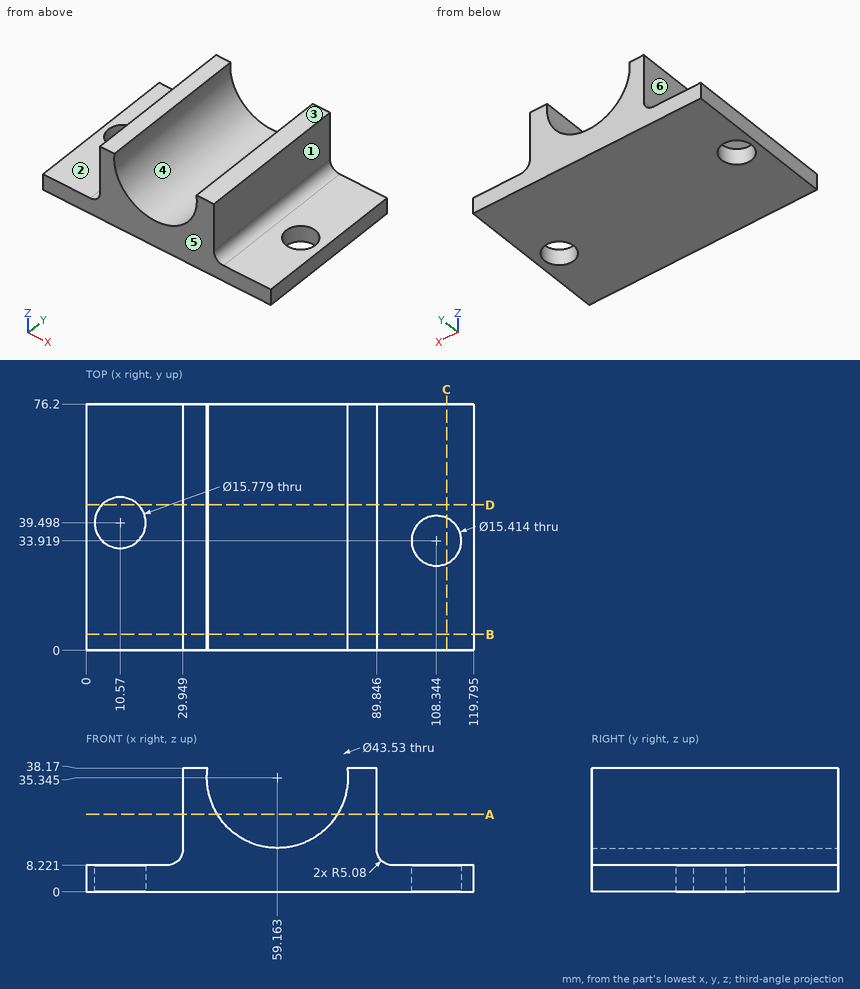
Study the drawing (mm; zero at the part's minimum x, y, z) and answer. A direction names the side the tool comes from. Give positions to 0.01 mm unless a question says otherwise; leave off trailing zeros. Loops run counter-clockwise (first coordinate to the right, second up) from the corner with the lowest first, then second, coordinate; pieces in that order, holes last. Notation, with made-up numbers: (37, 61) - (58, 61) arc R23 cw to (58, 86) - close; hole circle Ø2 at (51, 3.25). An arc over 180 degrees is marked (long way). Answer as CSV lines item,"result". Start each with the question number.
1) Straight lines are drawn through the part: L1, parallel to X at y = 26, z = 34.5 (1 decimal); L2, parallel to Z at x = 20, y = 40; L3, parallel to Z at x = 75.5, y = 70 (1 decimal). For each, find the intervals that lie inside material, in ascending order. Write a range as from..to.
2) Find section B-B (y = 5). Write down the section's boundary in (x, z) (1 decimal), then the cut area to 3 significant figures.
3) Find section D-D (y = 45). Write down the section's boundary in (x, z) (1 decimal).
4) Determine the mould class of the marked faces 4, 5 and 6 for opening direction X: released by +X, released by -X, zero draft, split by the parting line, or undercut.
5) Which of the six approach directions +Z, -Z, +X, -X, +Y, -Y give full straight-line access (tool end or side, diameter ignored) to the marked faces 1, 2 and 3?
6) Find section C-C (x = 111.5). Write down the section's boundary in (y, z).
7) Find section A-A (z = 24). Write down the section's boundary in (x, y).
8) Each of these flat-tipped pins is pushed along its axis until it touches: pin 1 Ø12.5 at (x, y) = (108.5, 29) entering from +Z; pin 2 Ø8 at (x, y) = (62.5, 20) entering from +Z (1 decimal); pin 3 Ø1 at (y, z) = (57, 21) entering from +X. Where does it stop, or does it pass through?
Findings below:
1,L1,"29.9..37.4, 80.9..89.8"
1,L2,"0..8.22"
1,L3,"0..21"
2,outline,"(0, 0) - (119.8, 0) - (119.8, 8.2) - (94.9, 8.2) arc R5.1 cw to (89.8, 13.3) - (89.8, 38.2) - (80.7, 38.2) arc R21.8 cw (long way) to (37.6, 38.2) - (29.9, 38.2) - (29.9, 13.3) arc R5.1 cw to (24.9, 8.2) - (0, 8.2) - close"
2,area,"1,920 mm^2"
3,outline,"(0, 0) - (4.9, 0) - (4.9, 8.2) - (0, 8.2) - close; (16.2, 0) - (119.8, 0) - (119.8, 8.2) - (94.9, 8.2) arc R5.1 cw to (89.8, 13.3) - (89.8, 38.2) - (80.7, 38.2) arc R21.8 cw (long way) to (37.6, 38.2) - (29.9, 38.2) - (29.9, 13.3) arc R5.1 cw to (24.9, 8.2) - (16.2, 8.2) - close"
4,face 4,"undercut"
4,face 5,"zero draft"
4,face 6,"released by -X"
5,face 1,"+Z, +X, +Y, -Y"
5,face 2,"+Z, -X, +Y, -Y"
5,face 3,"+Z, +X, -X, +Y, -Y"
6,outline,"(0, 0) - (26.89, 0) - (26.89, 8.22) - (0, 8.22) - close; (40.95, 0) - (76.2, 0) - (76.2, 8.22) - (40.95, 8.22) - close"
7,outline,"(29.95, 0) - (40.59, 0) - (40.59, 76.2) - (29.95, 76.2) - close; (77.74, 0) - (89.85, 0) - (89.85, 76.2) - (77.74, 76.2) - close"
8,pin 1,"z = 8.22"
8,pin 2,"z = 14.9"
8,pin 3,"x = 89.85"
